```python
from build123d import *

# Parameters (mm, degrees)
DODANIE_WYCI_GNI_CIE1_DEPTH = 2
SZKIC4_W                    = 10
SZKIC4_H                    = 45
DODANIE_WYCI_GNI_CIE2_DEPTH = 3


with BuildPart() as part:
    # Szkic1 → Dodanie-wyciągnięcie1 (new body)
    with BuildSketch(Plane(origin=(0, 0, 0), x_dir=(1, 0, 0), z_dir=(0, 1, 0))):
        Polygon((-21.15, 7.5), (-12, 7.5), (-12, -2.5), (12, -2.5), (12, 7.5), (21.15, 7.5), (21.15, -7.5), (-21.15, -7.5), align=None)
        with BuildLine():
            Line((-14, 2.5), (-14, -2.5))
            ThreePointArc((-14, -2.5), (-15.5, -4), (-17, -2.5))
            Line((-17, -2.5), (-17, 2.5))
            ThreePointArc((-17, 2.5), (-15.5, 4), (-14, 2.5))
        make_face(mode=Mode.SUBTRACT)
        with BuildLine():
            Line((17, 2.5), (17, -2.5))
            ThreePointArc((17, -2.5), (15.5, -4), (14, -2.5))
            Line((14, -2.5), (14, 2.5))
            ThreePointArc((14, 2.5), (15.5, 4), (17, 2.5))
        make_face(mode=Mode.SUBTRACT)
    extrude(amount=DODANIE_WYCI_GNI_CIE1_DEPTH)

    # Szkic4 → Dodanie-wyciągnięcie2 (add)
    with BuildSketch(Plane.XY.offset(7.5)):
        with Locations((0, 22.5)):
            Rectangle(SZKIC4_W, SZKIC4_H)
    extrude(amount=-DODANIE_WYCI_GNI_CIE2_DEPTH)


solid = part.part
```
Check sheet for the modelled part. Datum: model origin and axes. Units: mm. A direction names the side the tool comes from. Give positions to 0.01 mm unless a question says otherwise; leave off trailing zeros. Order: outer loops, then holes, each group sorted by start corner. A loop starts at its lowest first (then second) coordinate and runs counter-clockwise, first axis right, second up. Notation, with made-up numbers: M 63,60 L 101,60 A23 ccw 101,97 Z; hole C 26,85.5 d11. An arc over 180 degrees is marked long. Answer in a Markdown table with one row per item.
1) Thickness scan on L1, parallel to Z at x = -2.5, y = 25; L2, parallel to Y at x = 5.5, z = 5; L3, parallel to X at y = 32, z = 5.5. Record the ranges inside material, lowest first. Write a range as [from, to].
Filled sheet:
| item | result |
|---|---|
| L1 | z = [4.5, 7.5] |
| L2 | y = [0, 2] |
| L3 | x = [-5, 5] |
2) Access from +Z, -Z, +X, -X, +Y, -Y to the whole of each face (thin tool, end or side, straight path). Record for faces 1 (the flat face through (-5, 23, 6)), 2 (the flat face through (0, 1, 2.5)), 3 (the cylindrical face through (15.5, 1, -4)), 4 (the flat face through (5, 23, 6)).
Filled sheet:
| item | result |
|---|---|
| face 1 | +Z, -Z, -X, +Y |
| face 2 | -Z, +Y, -Y |
| face 3 | +Y, -Y |
| face 4 | +Z, -Z, +X, +Y |
3) Gauge pin test, flat ends, axial feed: P1, Ø1.5, axis at y = 31, z = 6, coming from the -X side; P2, Ø1.6, axis at x = -5, y = 1, coming from the -Z side; P3, Ø6, axis at x = 1.5, z = 3, coming from the +Y side; P4, Ø4, axis at x = -2.5, y = 7, coming from the -Z side. Record the tip position at first contact, or that the pin passes through.
Filled sheet:
| item | result |
|---|---|
| P1 | stops at x = -5 |
| P2 | stops at z = 2.5 |
| P3 | stops at y = 45 |
| P4 | stops at z = 4.5 |
4) Cross-section at D-D, the plane x = 11. Enter the section's corners in (y, z).
Filled sheet:
| item | result |
|---|---|
| outline | M 0,2.5 L 2,2.5 L 2,7.5 L 0,7.5 Z |
5) Cross-section at C-C, the plane y = 38. Enter the section's corners in (x, z).
Filled sheet:
| item | result |
|---|---|
| outline | M -5,4.5 L 5,4.5 L 5,7.5 L -5,7.5 Z |
6) Release check for a two-part mould opening along Z. For faces 5 (the flat face through (17, 1, 0)), 6 (the flat face through (17, 1, -7.5)), 7 (the flat face through (-12, 1, -3)) record: +Z half, -Z half, draft (parallel to the pull), parting line (faces both ways), or undercut.
Filled sheet:
| item | result |
|---|---|
| face 5 | undercut |
| face 6 | -Z half |
| face 7 | draft |
7) Cross-section at B-B, the plane x = -15.5. Enter the section's corners in (y, z), plus the area to 3 significant figures.
Filled sheet:
| item | result |
|---|---|
| outline | M 0,-7.5 L 2,-7.5 L 2,-4 L 0,-4 Z; M 0,4 L 2,4 L 2,7.5 L 0,7.5 Z |
| area | 14.0 mm2 |
8) Cross-section at A-A, the plane z = -6.5. Enter the section's corners in (x, y).
Filled sheet:
| item | result |
|---|---|
| outline | M -21.15,0 L -12,0 L -12,2 L -21.15,2 Z; M 12,0 L 21.15,0 L 21.15,2 L 12,2 Z |
